from build123d import *

# Parameters (mm, degrees)
SKETCH1_W           = 6.35
SKETCH1_H           = 33.02
BOSS_EXTRUDE1_DEPTH = 190.5
SKETCH3_R           = 2.54
CUT_EXTRUDE2_DEPTH  = 194.444805823


with BuildPart() as part:
    # Sketch1 → Boss-Extrude1 (new body)
    with BuildSketch(Plane.XY):
        with Locations((-3.175, 16.51)):
            Rectangle(SKETCH1_W, SKETCH1_H)
    extrude(amount=-BOSS_EXTRUDE1_DEPTH)

    # Sketch3 → Cut-Extrude2 (cut, through all)
    with BuildSketch(Plane(origin=(0, 33.02, 0), x_dir=(1, 0, 0), z_dir=(0, 1, 0))):
        with Locations(Location((-3.175, 6.35, 0), (0, 0, 270))):
            Circle(SKETCH3_R)
        with Locations(Location((-3.175, 184.15, 0), (0, 0, 270))):
            Circle(SKETCH3_R)
    extrude(amount=-CUT_EXTRUDE2_DEPTH, mode=Mode.SUBTRACT)


solid = part.part
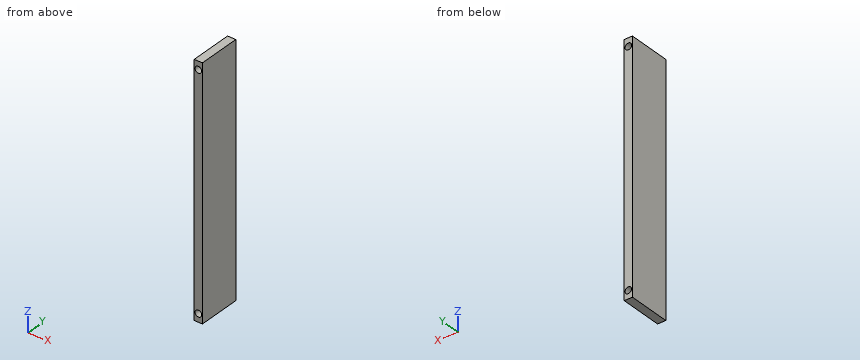
The listing builds one solid part. Answer for the finished solid, in the listing's coordinates (mm). Round coordinates to 2 decimals unless told otherwise and drop trailing zeros. Order: outer loops, then holes, each group sorted by start corner. A loop starts at its lowest first (then second) coordinate and runs counter-clockwise, first axis right, second up. Notation, with made-up numbers: (53, -38) -> (72, -38) arc R20 cw to (72, -23) -> close; hole circle Ø10 at (34.5, 79.5). An arc over 180 degrees is marked (long way). Write each question's results on one line, items separated by ' | '. Start each with the question number.
Q1. Find section C-C (y = 11.5). Determine the outline of the cut face in (x, z) (3 decimals), then the cut area to 3 significant figures.
Q2. Find section A-A (z = -184.15). Determine the outline of the cut face in (x, y) (3 decimals), then the cut area to 3 significant figures.
Q3. Straight lines are drawn through the part: probe 1 along Z at (x, y) = (-3.25, 4.5); probe 2 along X at (y, z) = (14, -184); probe 3 along Z at (x, y) = (-1, 20.5). For each, find the intervals that lie inside material, in ascending order. Write a range as from..to.
Q4. Find section B-B (x = -2). Determine the outline of the cut face in (y, z).
Worked answers:
1) outline: (-6.35, -190.5) -> (0, -190.5) -> (0, 0) -> (-6.35, 0) -> close; hole circle Ø5.08 at (-3.175, -184.15); hole circle Ø5.08 at (-3.175, -6.35) | area: 1,170 mm2
2) outline: (-6.35, 0) -> (-5.715, 0) -> (-5.715, 33.02) -> (-6.35, 33.02) -> close; (-0.635, 0) -> (0, 0) -> (0, 33.02) -> (-0.635, 33.02) -> close | area: 41.9 mm2
3) probe 1: z = -190.5..-186.69, -181.61..-8.89, -3.81..0 | probe 2: x = -6.35..-5.71, -0.64..0 | probe 3: z = -190.5..-185.46, -182.84..-7.66, -5.04..0
4) outline: (0, -190.5) -> (33.02, -190.5) -> (33.02, -186.4) -> (0, -186.4) -> close; (0, -181.9) -> (33.02, -181.9) -> (33.02, -8.6) -> (0, -8.6) -> close; (0, -4.1) -> (33.02, -4.1) -> (33.02, 0) -> (0, 0) -> close
